Build history of the part. All positions in model axes, mm. Face numbers are marked on the shaded views. A direction names the side the tool comes from. Round coordinates to 2 decimals unless told otherwise and drop trailing zeros. Order: outer loops, then holes, each group sorted by start corner. A loop starts at its lowest first (then second) coordinate and runs counter-clockwise, first axis right, second up. Notation, with made-up numbers: (55.5, 37) -> (93.5, 37) arc R27 ccw to (93.5, 55) -> close; hole circle Ø2 at (23.25, -7). An arc over 180 degrees is marked (long way). Answer as CSV lines item,"result". Start each with the question number.
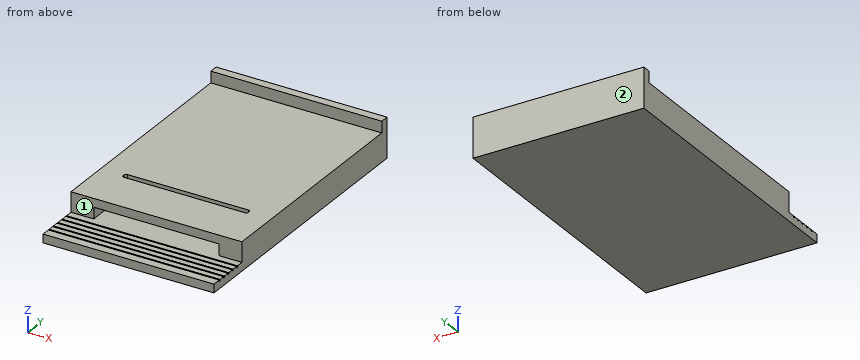
```python
from build123d import *

# Parameters (mm, degrees)
F0_W      = 381
F0_H      = 609.6
F1_DEPTH  = 19.05
F2_W      = 50.8
F2_H      = 457.2
F3_DEPTH  = 25.4
F4_W      = 381
F4_H      = 508
F5_DEPTH  = 19.05
F6_W      = 381
F6_H      = 88.9
F7_DEPTH  = 19.05
F8_W      = 3.175
F8_H      = 3.175
F9_DEPTH  = 381
F10_W     = 279.4
F10_H     = 12.7
F11_DEPTH = 19.05
F12_R     = 5.08


with BuildPart() as f1:
    # F0 (on Top) → F1 (new body)
    with BuildSketch(Plane.XY):
        with Locations((-190.5, 304.8)):
            Rectangle(F0_W, F0_H)
    extrude(amount=F1_DEPTH)

    # F2 (on face) → F3 (join)
    with BuildSketch(Plane.XY.offset(19.05)):
        with Locations((-25.4, 330.2)):
            Rectangle(F2_W, F2_H)
        Polygon((0, 609.6), (-381, 609.6), (-381, 558.8), (-330.2, 558.8), (-50.8, 558.8), (0, 558.8), align=None)
        with Locations((-355.6, 330.2)):
            Rectangle(F2_W, F2_H)
    extrude(amount=F3_DEPTH)

    # F4 (on face) → F5 (join)
    with BuildSketch(Plane.XY.offset(44.45)):
        with Locations((-190.5, 355.6)):
            Rectangle(F4_W, F4_H)
    extrude(amount=F5_DEPTH)

    # F6 (on face) → F7 (join)
    with BuildSketch(Plane(origin=(0, 609.6, 0), x_dir=(-1, 0, 0), z_dir=(0, 1, 0))):
        with Locations((190.5, 44.45)):
            Rectangle(F6_W, F6_H)
    extrude(amount=F7_DEPTH)

    # F8 (on face) → F9 (cut)
    with BuildSketch(Plane.YZ):
        with Locations((20.6375, 17.4625)):
            Rectangle(F8_W, F8_H)
        with Locations((36.5125, 17.4625)):
            Rectangle(F8_W, F8_H)
        with Locations((52.3875, 17.4625)):
            Rectangle(F8_W, F8_H)
        with Locations((68.2625, 17.4625)):
            Rectangle(F8_W, F8_H)
        with Locations((84.1375, 17.4625)):
            Rectangle(F8_W, F8_H)
    extrude(amount=-F9_DEPTH, mode=Mode.SUBTRACT)

    # F10 (on face) → F11 (cut)
    with BuildSketch(Plane.XY.offset(63.5)):
        with Locations((-190.5, 209.55)):
            Rectangle(F10_W, F10_H)
    extrude(amount=-F11_DEPTH, mode=Mode.SUBTRACT)

    # F12
    f12_edges = [f1.edges().sort_by_distance(p)[0] for p in [
        (-330.2, 215.9, 53.975),
        (-330.2, 203.2, 53.975),
        (-50.8, 215.9, 53.975),
        (-50.8, 203.2, 53.975),
    ]]
    fillet(f12_edges, radius=F12_R)


solid = f1.part
```
Q1. Slice it at B-B, the plane z = 51.5. Write the cut outline in (x, y), plus the area to 3 significant figures.
Q2. Flat gauge pins, fed straight in: pin 1 Ø1 at (x, y) = (-137, 67.5) entering from +Z (3 decimals); pin 2 Ø2.5 at (x, y) = (-203, 53) entering from +Z; pin 3 Ø8 at (x, z) = (-304.5, 73) entering from -Y. Where does each tip first touch, or does it go through?
Q3. Which spindle directions (+Z, -Z, +X, -X, +Y, -Y) get a long thin tool onto all of the face, cutting with end or side? Do the marked faces 1 and 2. Say none if no direction does.
Q4. Slice it at C-C, the plane y = 549. Write the cut outline in (x, z).
Q5. Probe L1, parallel to X at y = 288, z = 34; L2, parallel to Z at x = -102.5, y = 268; L3, parallel to Y at x = -175.5, z = 29.5. List the from-to ranges inside material, lowest first.
Q6. Slice it at D-D, the plane z = 82. Write the cut outline in (x, y), plus the area to 3 significant figures.
Solutions:
1,outline,"(-381, 101.6) -> (0, 101.6) -> (0, 628.65) -> (-381, 628.65) -> close; hole (-330.2, 208.28) arc R5.08 ccw to (-325.12, 203.2) -> (-55.88, 203.2) arc R5.08 ccw to (-50.8, 208.28) -> (-50.8, 210.82) arc R5.08 ccw to (-55.88, 215.9) -> (-325.12, 215.9) arc R5.08 ccw to (-330.2, 210.82) -> close"
1,area,"197,000 mm2"
2,pin 1,"stops at z = 15.875"
2,pin 2,"stops at z = 19.05"
2,pin 3,"stops at y = 609.6"
3,face 1,"+Z, +X, -X, -Y"
3,face 2,"+Z, -Z, +X, -X, +Y"
4,outline,"(-381, 0) -> (0, 0) -> (0, 63.5) -> (-381, 63.5) -> close; hole (-330.2, 19.05) -> (-50.8, 19.05) -> (-50.8, 44.45) -> (-330.2, 44.45) -> close"
5,L1,"x = -381 to -330.2, -50.8 to 0"
5,L2,"z = 0 to 19.05, 44.45 to 63.5"
5,L3,"y = 558.8 to 628.65"
6,outline,"(-381, 609.6) -> (0, 609.6) -> (0, 628.65) -> (-381, 628.65) -> close"
6,area,"7,260 mm2"
